Here's the drawing with two shaded views (mm, measured from the low corner). I have some questions. A direction names the side the tool comes from. Round coordinates to 2 decimals unless told otherwise and drop trailing zeros.
Q1. We'd pull the mould along Z, two halves only. Please class the marked faces 3, 4, 5 and 6: pulls with the +Z half, pulls with the -Z half, needs draft (parallel to the pull), parting line crosses it, or undercut.
Q2. Will these pins go through, and if not, where does the flat tip stop? P1, Ø3, axis at x = 2.5, z = 7, coming from the -Y side (1 decimal); P2, Ø3, axis at x = 10.5, y = 3, coming from the +Z side; P3, Ø0.7, axis at x = 4, y = 0.5, coming from the +Z side.
Q3. For the marked faces 1 and 2, which set-ups out of +Z, -Z, +X, -X, +Y, -Y let a thin tool reach every point of the face, with its end or its side?
Q4. If I drill on line 1 (Z direction, x = 8, y = 4.25) (1 decimal); line 2 (Z direction, x = 11.75, y = 0.5) (1 decimal); line 3 (X direction, y = 5, z = 11.5) (1 decimal), over which ranges is the centre line in solid material (lowest first)?
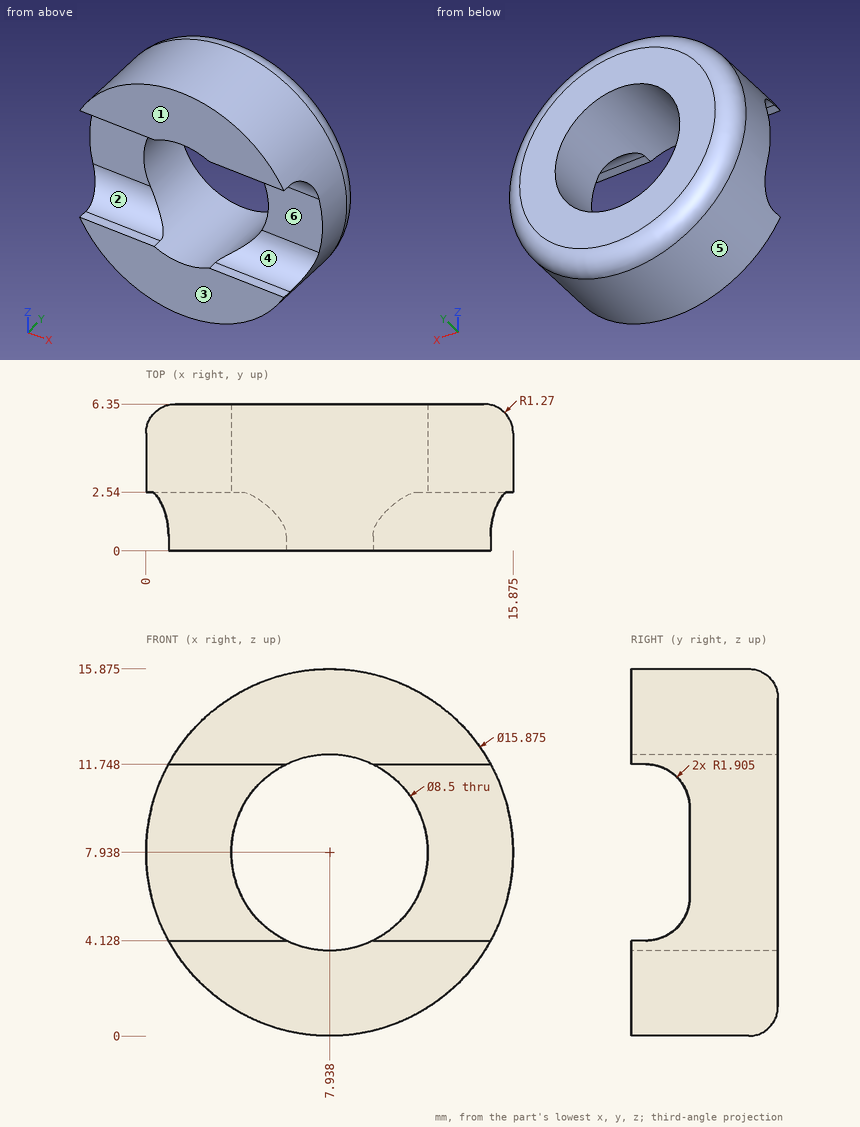
Solution:
1. face 3: needs draft
1. face 4: undercut
1. face 5: parting line crosses it
1. face 6: undercut
2. P1: stops at y = 2.5
2. P2: stops at z = 15.8
2. P3: stops at z = 15.02
3. face 1: +Z, -Z, +X, -X, -Y
3. face 2: +X, -X, -Y
4. line 1: z = 0 to 3.7, 12.2 to 15.9
4. line 2: z = 1 to 4.1, 11.7 to 14.9
4. line 3: x = 0.8 to 5.6, 10.3 to 15
